from build123d import *

# Parameters (mm, degrees)
PAD_DEPTH    = 4
SKETCH001_R  = 2
POCKET_DEPTH = 5
SKETCH002_R  = 1
PAD001_DEPTH = 3.5


with BuildPart() as part:
    # Sketch → Pad (new body)
    with BuildSketch(Plane.XY):
        Polygon((-10, 0), (0, 10), (10, 0), (10, -15), (0, -20), (-10, -15), align=None)
    extrude(amount=PAD_DEPTH)

    # Sketch001 (on Face8 of Pad) → Pocket (cut)
    with BuildSketch(Plane.XY.offset(4)):
        Circle(SKETCH001_R)
    extrude(amount=-POCKET_DEPTH, mode=Mode.SUBTRACT)

    # Sketch002 (on Face5 of Pocket) → Pad001 (join)
    with BuildSketch(Plane.XY.offset(4)):
        with Locations((0, 6.08)):
            Circle(SKETCH002_R)
        with Locations((-6.08, 0)):
            Circle(SKETCH002_R)
        with Locations((6.08, 0)):
            Circle(SKETCH002_R)
        with Locations((0, -6.08)):
            Circle(SKETCH002_R)
    extrude(amount=PAD001_DEPTH)

    # Sketch006 → Revolution (revolve)
    with BuildSketch(Plane.XZ):
        with BuildLine():
            ThreePointArc((-6.08, 9.5), (-7.198034, 8.809017), (-7.08, 7.5))
            Line((-7.08, 7.5), (-6.08, 7.5))
            Line((-6.08, 7.5), (-6.08, 9.5))
        make_face()
    revolve(axis=Axis((-6.08, 0, 7.5), (0, 0, 1)))

    # Sketch008 → Revolution001 (revolve)
    with BuildSketch(Plane.XZ):
        with BuildLine():
            ThreePointArc((7.08, 7.5), (7.198034, 8.809017), (6.08, 9.5))
            Line((6.08, 7.5), (6.08, 9.5))
            Line((7.08, 7.5), (6.08, 7.5))
        make_face()
    revolve(axis=Axis((6.08, 0, 7.5), (0, 0, 1)))


solid = part.part
Work out the finished part from the listing and answer in its coordinate system (mm). A direction names the side the tool comes from. Round coordinates to 2 decimals unless told otherwise and drop trailing zeros. Write each loop counter-clockwise with the first axis right and the second up, starting at its lowest first coordinate (ties: lowest second). Pieces come first, ordered by that corner, then holes. Notation, with made-up numbers: (29, 32) -> (76, 32) arc R10 ccw to (76, 48) -> close; hole circle Ø3 at (55, 75.25). An arc over 180 degrees is marked (long way). Answer as CSV lines item,"result". Start each with the question number.
(1) The part is cut by section B-B, the plane y = 6.08. Give the vertices of the cut face in (x, z), then the cut area to 3 significant figures.
(2) A tool of negligible diameter and unlimited length cuts with its end or side. For faces 1 (the cylindrical face through (-0.13, -5.09, 5.73)), 2 (the cylindrical face through (-7.08, 0.04, 5.73)), 3 (the flat face through (0, -6, 7.5)), from which of +Z, -Z, +X, -X, +Y, -Y can it reach the whole face along a straight path? Write none if from no direction.
(3) The part is cut by section A-A, the plane x = -6.08. Give the vertices of the cut face in (y, z).
(4) The part is cut by section D-D, the plane y = -15.5. Give the vertices of the cut face in (x, z).
(5) The mould has two halves that part along Z. Classify faces 4 (the cylindrical face through (7.034, 0.3, 5.726)), 5 (the flat face through (0, -5, 0)), 6 (the flat face through (5, 5, 2)): +Z half, -Z half, draft (parallel to the pull), parting line (faces both ways), or undercut.
(6) The part is cut by section C-C, the plane z = 6.5. Give the vertices of the cut face in (x, y).
(7) Each of these flat-tipped pins is pushed along its axis until it touches: pin 1 (4.5 mm diameter, centred on x = 0, y = 0, fed in from -Z); pin 2 (1.6 mm diameter, centred on x = 0.5, y = -5.5, fed in from +Z); pin 3 (1.5 mm diameter, centred on y = 1.5, z = 2, fed in from +X); pin 4 (2 mm diameter, centred on x = 4, y = -8.5, fed in from +Z). Where does it stop, or does it pass through?
(8) Find the intervals of material crossed by probe 1 along Z at (x, y) = (4.5, 4.75); probe 2 along Z at (x, y) = (-0.75, 6); probe 3 along X at (y, z) = (0.75, 5.25), in increasing order.
Output values:
1,outline,"(-3.92, 0) -> (3.92, 0) -> (3.92, 4) -> (1, 4) -> (1, 7.5) -> (-1, 7.5) -> (-1, 4) -> (-3.92, 4) -> close"
1,area,"38.4 mm²"
2,face 1,"+Z"
2,face 2,"none"
2,face 3,"+Z, +X, -X, +Y, -Y"
3,outline,"(-16.96, 0) -> (3.92, 0) -> (3.92, 4) -> (1, 4) -> (1, 7.5) arc R1.25 ccw (long way) to (-1, 7.5) -> (-1, 4) -> (-16.96, 4) -> close"
4,outline,"(-9, 0) -> (9, 0) -> (9, 4) -> (-9, 4) -> close"
5,face 4,"undercut"
5,face 5,"-Z half"
5,face 6,"draft"
6,outline,"circle Ø2 at (-6.08, 0); circle Ø2 at (0, -6.08); circle Ø2 at (0, 6.08); circle Ø2 at (6.08, 0)"
7,pin 1,"stops at z = 0"
7,pin 2,"stops at z = 7.5"
7,pin 3,"stops at x = 9.25"
7,pin 4,"stops at z = 4"
8,probe 1,"z = 0 to 4"
8,probe 2,"z = 0 to 7.5"
8,probe 3,"x = -6.74 to -5.42, 5.42 to 6.74"
